from build123d import *

# Parameters (mm, degrees)
F0_W     = 2.75
F0_H     = 5.5
F1_DEPTH = 95
F2_R     = 2
F3_R     = 0.25
F4_DEPTH = 5
F5_DEPTH = 5


with BuildPart() as f1:
    # F0 (on Front) → F1 (new body)
    with BuildSketch(Plane.XZ):
        with Locations((1.375, 2.75)):
            Rectangle(F0_W, F0_H)
        Polygon((0, 0), (-2.75, 0), (-2.75, -2.5), (-6.75, -2.5), (-6.75, -7.5), (6.75, -7.5), (6.75, -2.5), (2.75, -2.5), (2.75, 0), align=None)
        Polygon((2.75, 5.5), (2.75, 0), (6.75, 0), align=None)
        with Locations((-1.375, 2.75)):
            Rectangle(F0_W, F0_H)
        Polygon((-2.75, 5.5), (-6.75, 0), (-2.75, 0), align=None)
    extrude(amount=F1_DEPTH)

    # F2
    f2_edges = [f1.edges().sort_by_distance(p)[0] for p in [
        (2.75, -47.5, 5.5),
        (-2.75, -47.5, 5.5),
    ]]
    fillet(f2_edges, radius=F2_R)

    # F3
    f3_edges = [f1.edges().sort_by_distance(p)[0] for p in [
        (6.75, -47.5, 0),
        (-6.75, -47.5, 0),
    ]]
    fillet(f3_edges, radius=F3_R)

    # F4 (add): a face of the model
    f4_faces = [f1.faces().sort_by_distance(p)[0] for p in [
        (-6.75, -47.5, -5),
    ]]
    extrude(f4_faces, amount=F4_DEPTH)

    # F5 (add): a face of the model
    f5_faces = [f1.faces().sort_by_distance(p)[0] for p in [
        (6.75, -47.5, -5),
    ]]
    extrude(f5_faces, amount=F5_DEPTH)


solid = f1.part
The model under review builds one solid part; all positions refer to its coordinate system, in mm. A direction names the side the tool comes from. Round coordinates to 2 decimals unless told otherwise and drop trailing zeros. Loops run counter-clockwise (first coordinate to the right, second up) from the corner with the lowest first, then second, coordinate; pieces in that order, holes last. Notation, with made-up numbers: (32.25, 15.25) -> (66.25, 15.25) arc R12 cw to (66.25, 28.25) -> close; hole circle Ø2 at (36, 34). An arc over 180 degrees is marked (long way). Write item = value, one per line. Start each with the question number.
Item 1: Take a section at A-A on y = -14.5. Give the boundary of the cut face in (x, z), plus the area to 3 significant figures.
Item 2: Take a section at C-C on z = 3.25. Give the boundary of the cut face in (x, y).
Item 3: To check wall thickness, follow L1, parallel to Z at x = -7.75, y = -22; L2, parallel to X at y = -13, z = -1.5; L3, parallel to Z at x = 4, y = -4. State the ranges of each line that lie inside material, in increasing order.
Item 4: Take a section at B-B on x = 9. Give the boundary of the cut face in (y, z).
Item 5: Insertion check: pin 1 (2.5 mm diameter, centred on x = 6, y = -69.5, fed in from +Z); pin 2 (5 mm diameter, centred on y = -12.5, z = 2, fed in from -X); pin 3 (3 mm diameter, centred on x = -7, y = -52.5, fed in from +Z). Each pin has a flat end and moves straight along its axis. Give the tip position at first contact, or say it passes through.
Item 6: Mouldability with a two-part tool opening along Z and no side actions: class faces 1 (the flat face through (-4.88, -46.84, 2.57)), 2 (the flat face through (-11.75, -47, -5)), 3 (the flat face through (2.75, -47, -1)) as released by +Z, released by -Z, zero draft, split by the parting line, or undercut.
Item 7: For faces 4 (the flat face through (4, -47, 0)), 5 (the cylindrical face through (-2.6, -48.2, 5.3)), 6 (the flat face through (-2.75, -47, -1)), list the 3-axis set-ups (+Z, -Z, +X, -X, +Y, -Y) from which the entire face can be reached by the end or side of a thin tool; tool diameter is ignored.
Result:
q1.outline = (-11.75, -7.5) -> (11.75, -7.5) -> (11.75, -2.5) -> (2.75, -2.5) -> (2.75, 0) -> (6.26, 0) arc R0.25 ccw to (6.46, 0.4) -> (3.35, 4.68) arc R2 ccw to (1.73, 5.5) -> (-1.73, 5.5) arc R2 ccw to (-3.35, 4.68) -> (-6.46, 0.4) arc R0.25 ccw to (-6.26, 0) -> (-2.75, 0) -> (-2.75, -2.5) -> (-11.75, -2.5) -> close
q1.area = 183 mm²
q2.outline = (-4.39, -95) -> (4.39, -95) -> (4.39, 0) -> (-4.39, 0) -> close
q3.L1 = -7.5 to -2.5
q3.L2 = -2.75 to 2.75
q3.L3 = -7.5 to -2.5, 0 to 3.78
q4.outline = (-95, -7.5) -> (0, -7.5) -> (0, -2.5) -> (-95, -2.5) -> close
q5.pin_1 = 2.75
q5.pin_2 = -6.51
q5.pin_3 = 1.72
q6.face_1 = released by +Z
q6.face_2 = zero draft
q6.face_3 = undercut
q7.face_4 = +X, +Y, -Y
q7.face_5 = +Z, -X, +Y, -Y
q7.face_6 = -X, +Y, -Y
